Read the model definition and answer for the solid it produces. Units are mm, in the model's axes. Round coordinates to 2 decimals unless told otherwise and drop trailing zeros. Order: outer loops, then holes, each group sorted by start corner. A loop starts at its lowest first (then second) coordinate and runs counter-clockwise, first axis right, second up. Notation, with made-up numbers: (18.5, 80.25) - (37.5, 80.25) arc R16 cw to (37.5, 92.25) - close; hole circle Ø9 at (10, 39.25). An arc over 180 degrees is marked (long way). Put each result on its own line as item: value. Start each with the question number.
Q1. Section D-D on x = 39 is taken. State how many separate pieces and enclosed holes the cut face has, then the cut area to 3 significant figures.
Q2. Each of these flat-tipped pins is pushed along its axis until it touches: pin 1 Ø12 at (x, z) = (34, 22) entering from +Y; pin 2 Ø1.5 at (y, z) = (-3, 93.5) entering from -X; pin 3 Ø4 at (y, z) = (-3.5, 72) entering from +X; pin 4 Ø4 at (x, z) = (81.5, 84) entering from -Y. Where does it stop, or does it pass through?
Q3. Find the intervals of material crossed by line 1 along Z through (x, y) = (-5, -11.5); line 2 along Y through (x, z) = (91.5, 19.5); line 3 along Z through (x, y) = (24, -11.5), in increasing order. Write a range as from..to.
Q4. Section C-C on z = 7.5 is taken. Give the vertices of the cut face in (x, y), then the cut area to 3 significant figures.
Q5. Section B-B on x = -5 is taken. Give the vertices of the cut face in (y, z), then the cut area to 3 significant figures.
Q6. Section A-A on y = -10.75 is taken. Give the vertices of the cut face in (x, z).
from build123d import *

# Parameters (mm, degrees)
F0_W      = 149
F0_H      = 145
F0_W_2    = 19
F0_H_2    = 20
F0_H_3    = 15
F1_DEPTH  = 5
F2_W      = 149
F2_H      = 15
F3_DEPTH  = 10
F4_W      = 7.5
F4_H      = 15
F5_DEPTH  = 10
F6_R      = 3
F7_DEPTH  = 7.5
F9_DEPTH  = 10
F10_R     = 2.5
F11_DEPTH = 7.5


with BuildPart() as f1:
    # F0 (on Front) → F1 (new body)
    with BuildSketch(Plane.XZ):
        with Locations((74.5, 72.5)):
            Rectangle(F0_W, F0_H)
        with Locations((14.5, 30)):
            Rectangle(F0_W_2, F0_H_2, mode=Mode.SUBTRACT)
        with Locations((38.5, 30)):
            Rectangle(F0_W_2, F0_H_2, mode=Mode.SUBTRACT)
        with Locations((62.5, 30)):
            Rectangle(F0_W_2, F0_H_2, mode=Mode.SUBTRACT)
        with Locations((14.5, 52.5)):
            Rectangle(F0_W_2, F0_H_3, mode=Mode.SUBTRACT)
        with Locations((38.5, 52.5)):
            Rectangle(F0_W_2, F0_H_3, mode=Mode.SUBTRACT)
        with Locations((62.5, 52.5)):
            Rectangle(F0_W_2, F0_H_3, mode=Mode.SUBTRACT)
        with Locations((86.5, 30)):
            Rectangle(F0_W_2, F0_H_2, mode=Mode.SUBTRACT)
        with Locations((110.5, 30)):
            Rectangle(F0_W_2, F0_H_2, mode=Mode.SUBTRACT)
        with Locations((134.5, 30)):
            Rectangle(F0_W_2, F0_H_2, mode=Mode.SUBTRACT)
        with Locations((86.5, 52.5)):
            Rectangle(F0_W_2, F0_H_3, mode=Mode.SUBTRACT)
        with Locations((110.5, 52.5)):
            Rectangle(F0_W_2, F0_H_3, mode=Mode.SUBTRACT)
        with Locations((134.5, 52.5)):
            Rectangle(F0_W_2, F0_H_3, mode=Mode.SUBTRACT)
        with Locations((14.5, 72.5)):
            Rectangle(F0_W_2, F0_H_3, mode=Mode.SUBTRACT)
        with Locations((14.5, 92.5)):
            Rectangle(F0_W_2, F0_H_3, mode=Mode.SUBTRACT)
        with Locations((38.5, 72.5)):
            Rectangle(F0_W_2, F0_H_3, mode=Mode.SUBTRACT)
        with Locations((62.5, 72.5)):
            Rectangle(F0_W_2, F0_H_3, mode=Mode.SUBTRACT)
        with Locations((38.5, 92.5)):
            Rectangle(F0_W_2, F0_H_3, mode=Mode.SUBTRACT)
        with Locations((62.5, 92.5)):
            Rectangle(F0_W_2, F0_H_3, mode=Mode.SUBTRACT)
        with Locations((14.5, 112.5)):
            Rectangle(F0_W_2, F0_H_3, mode=Mode.SUBTRACT)
        with Locations((14.5, 132.5)):
            Rectangle(F0_W_2, F0_H_3, mode=Mode.SUBTRACT)
        with Locations((38.5, 112.5)):
            Rectangle(F0_W_2, F0_H_3, mode=Mode.SUBTRACT)
        with Locations((62.5, 112.5)):
            Rectangle(F0_W_2, F0_H_3, mode=Mode.SUBTRACT)
        with Locations((38.5, 132.5)):
            Rectangle(F0_W_2, F0_H_3, mode=Mode.SUBTRACT)
        with Locations((62.5, 132.5)):
            Rectangle(F0_W_2, F0_H_3, mode=Mode.SUBTRACT)
        with Locations((86.5, 72.5)):
            Rectangle(F0_W_2, F0_H_3, mode=Mode.SUBTRACT)
        with Locations((110.5, 72.5)):
            Rectangle(F0_W_2, F0_H_3, mode=Mode.SUBTRACT)
        with Locations((86.5, 92.5)):
            Rectangle(F0_W_2, F0_H_3, mode=Mode.SUBTRACT)
        with Locations((110.5, 92.5)):
            Rectangle(F0_W_2, F0_H_3, mode=Mode.SUBTRACT)
        with Locations((134.5, 72.5)):
            Rectangle(F0_W_2, F0_H_3, mode=Mode.SUBTRACT)
        with Locations((134.5, 92.5)):
            Rectangle(F0_W_2, F0_H_3, mode=Mode.SUBTRACT)
        with Locations((86.5, 112.5)):
            Rectangle(F0_W_2, F0_H_3, mode=Mode.SUBTRACT)
        with Locations((110.5, 112.5)):
            Rectangle(F0_W_2, F0_H_3, mode=Mode.SUBTRACT)
        with Locations((86.5, 132.5)):
            Rectangle(F0_W_2, F0_H_3, mode=Mode.SUBTRACT)
        with Locations((110.5, 132.5)):
            Rectangle(F0_W_2, F0_H_3, mode=Mode.SUBTRACT)
        with Locations((134.5, 112.5)):
            Rectangle(F0_W_2, F0_H_3, mode=Mode.SUBTRACT)
        with Locations((134.5, 132.5)):
            Rectangle(F0_W_2, F0_H_3, mode=Mode.SUBTRACT)
    extrude(amount=F1_DEPTH)

    # F2 (on face) → F3 (join)
    with BuildSketch(Plane.XZ.offset(5)):
        with Locations((74.5, 7.5)):
            Rectangle(F2_W, F2_H)
    extrude(amount=F3_DEPTH)

    # F4 (on face) → F5 (join)
    with BuildSketch(Plane(origin=(0, 0, 0), x_dir=(0, -1, 0), z_dir=(-1, 0, 0))):
        with Locations((11.25, 7.5)):
            Rectangle(F4_W, F4_H)
    extrude(amount=F5_DEPTH)

    # F6 (on face) → F7 (cut, through all)
    with BuildSketch(Plane(origin=(0, -7.5, 0), x_dir=(-1, 0, 0), z_dir=(0, 1, 0))):
        with Locations((5, 7.5)):
            Circle(F6_R)
    extrude(amount=-F7_DEPTH, mode=Mode.SUBTRACT)

    # F8 (on face) → F9 (join)
    with BuildSketch(Plane.YZ.offset(149)):
        Polygon((-7.5, 15), (-7.5, 0), (0, 0), (0, 15), (-5, 15), align=None)
    extrude(amount=F9_DEPTH)

    # F10 (on face) → F11 (join)
    with BuildSketch(Plane.XZ.offset(7.5)):
        with Locations((154, 7.5)):
            Circle(F10_R)
    extrude(amount=F11_DEPTH)


solid = f1.part
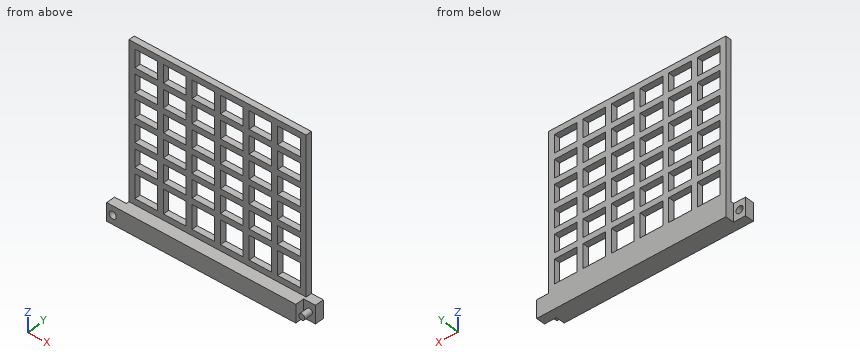
Findings:
1. separate pieces: 7
1. enclosed holes: 0
1. area: 400 mm2
2. pin 1: y = 0
2. pin 2: x = 0
2. pin 3: x = 149
2. pin 4: y = -5
3. line 1: 0..4.5, 10.5..15
3. line 2: -5..0
3. line 3: 0..15
4. outline: (-10, -15) - (-8, -15) - (-8, -7.5) - (-10, -7.5) - close; (-2, -15) - (149, -15) - (149, -7.5) - (151.5, -7.5) - (151.5, -15) - (156.5, -15) - (156.5, -7.5) - (159, -7.5) - (159, 0) - (0, 0) - (0, -7.5) - (-2, -7.5) - close
4. area: 2,380 mm2
5. outline: (-15, 0) - (-7.5, 0) - (-7.5, 4.5) - (-15, 4.5) - close; (-15, 10.5) - (-7.5, 10.5) - (-7.5, 15) - (-15, 15) - close
5. area: 67.5 mm2
6. outline: (-10, 0) - (149, 0) - (149, 15) - (-10, 15) - close; circle Ø5 at (154, 7.5); hole circle Ø6 at (-5, 7.5)
